For this review, take the finished solid that the model builds, in its own axes (mm). Face numbers are marked on the shaded views. A direction names the side the tool comes from. Coordinates: 2 decimals unless noted, no trailing zeros. Write each loop counter-clockwise with the first axis right and the second up, starting at its lowest first coordinate (ties: lowest second). Pieces come first, ordered by that corner, then holes. Notation, with made-up numbers: (47.5, -10) -> (71.5, -10) arc R27 ccw to (71.5, 18) -> close; hole circle Ø2 at (83.5, 70). An arc over 180 degrees is marked (long way). One line per item, written item: value. Start each with the question number.
1) Mouldability with a two-part tool opening along Y and no side actions: class the marked faces 1 and 2 as released by +Y, released by -Y, zero draft, split by the parting line, or undercut.
2) Add section B-B (z = 58). State the section outline as (x, y) points, and give its area (3 significant figures).
3) Machinability: for the marked faces 3 and 4, which of the approach directions +Z, -Z, +X, -X, +Y, -Y give a long, thin tool a straight path to every point of the face, cutting with its end or side? Answer none if there is none.
4) For pin 1 Ø6.5 at (x, z) = (0, 40.5) entering from -Y; pin 2 Ø3 at (x, z) = (-3, 58) entering from +Y; pin 3 Ø6 at (y, z) = (-4.5, 42.5) entering from -X; pin 4 Ø16 at (x, y) = (0, 0) entering from -Z, all flat-tipped, find the tip position at first contact; note any pin that passes through.
5) Add section A-A (x = 0). State the section outline as (y, z) points, and give its area (3 significant figures).
6) For probe 1 along Z at (x, y) = (1, -11); probe 2 along Y at (x, z) = (0, 68); probe 3 along Z at (x, y) = (0, 10.85), list the stretches that pass through material, from the lowest coordinate up. Write a range as from..to.
7) Add section D-D (x = 4). State the section outline as (y, z) points.
8) Add section C-C (y = 14). State the section outline as (x, z) points, and give its area (3 significant figures).
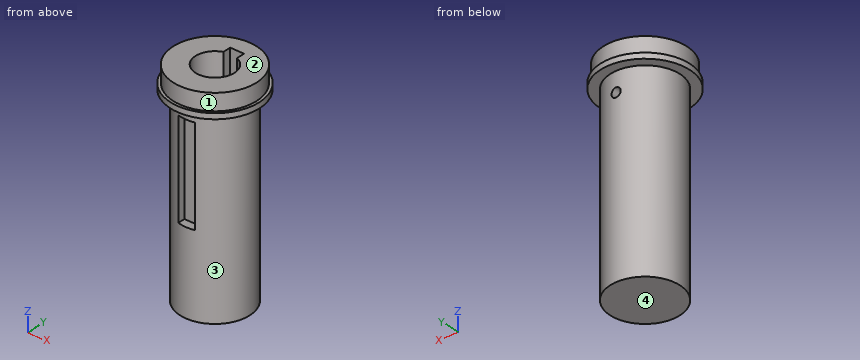
from build123d import *

# Parameters (mm, degrees)
SKETCH1_R                 = 12.5
BOSS_EXTRUDE1_DEPTH       = 68.7
SKETCH2_R                 = 16
BOSS_EXTRUDE2_DEPTH       = 2
SKETCH3_R                 = 15
BOSS_EXTRUDE3_DEPTH       = 6
CUT_EXTRUDE1_DEPTH        = 30
SKETCH6_W                 = 6
SKETCH6_H                 = 6
CUT_EXTRUDE2_DEPTH        = 35
M4X0_7_TAPPED_HOLE1_D     = 3.3
M4X0_7_TAPPED_HOLE1_DEPTH = 3


with BuildPart() as part:
    # Sketch1 → Boss-Extrude1 (new body)
    with BuildSketch(Plane.XY):
        Circle(SKETCH1_R)
    extrude(amount=BOSS_EXTRUDE1_DEPTH)

    # Sketch2 → Boss-Extrude2 (add)
    with BuildSketch(Plane.XY.offset(68.7)):
        Circle(SKETCH2_R)
    extrude(amount=BOSS_EXTRUDE2_DEPTH)

    # Sketch3 → Boss-Extrude3 (add)
    with BuildSketch(Plane.XY.offset(70.7)):
        Circle(SKETCH3_R)
    extrude(amount=BOSS_EXTRUDE3_DEPTH)

    # Sketch4 → Cut-Extrude1 (cut)
    with BuildSketch(Plane.XY.offset(76.7)):
        with BuildLine():
            Line((-2.5, 6.538348415), (-2.5, 4.5))
            Line((-2.5, 4.5), (2.5, 4.5))
            Line((2.5, 4.5), (2.5, 6.538348415))
            ThreePointArc((2.5, 6.538348415), (0, 7), (-2.5, 6.538348415))
        make_face()
        with BuildLine():
            Line((2.5, 4.5), (-2.5, 4.5))
            Line((-2.5, 4.5), (-2.5, 6.538348415))
            ThreePointArc((-2.5, 6.538348415), (-3.968626967, -5.766281297), (7, 0))
            ThreePointArc((7, 0), (5.766281297, 3.968626967), (2.5, 6.538348415))
            Line((2.5, 6.538348415), (2.5, 4.5))
        make_face()
        with BuildLine():
            Line((-2.5, 9.5), (-2.5, 6.538348415))
            ThreePointArc((-2.5, 6.538348415), (0, 7), (2.5, 6.538348415))
            Line((2.5, 6.538348415), (2.5, 9.5))
            Line((2.5, 9.5), (-2.5, 9.5))
        make_face()
    extrude(amount=-CUT_EXTRUDE1_DEPTH, mode=Mode.SUBTRACT)

    # Sketch6 → Cut-Extrude2 (cut)
    with BuildSketch(Plane(origin=(0, 0, 64.7), x_dir=(-1, 0, 0), z_dir=(0, 0, -1))):
        with Locations((0, -12.5)):
            Rectangle(SKETCH6_W, SKETCH6_H)
    extrude(amount=CUT_EXTRUDE2_DEPTH, mode=Mode.SUBTRACT)

    # M4x0.7 Tapped Hole1
    with Locations(Plane(origin=(0, 12.5, 0), x_dir=(1, 0, 0), z_dir=(0, 1, 0))):
        with Locations((0, -61.7)):
            Hole(M4X0_7_TAPPED_HOLE1_D / 2, depth=M4X0_7_TAPPED_HOLE1_DEPTH)


solid = part.part
Numbers:
1. face 1: split by the parting line
1. face 2: zero draft
2. outline: (-3, -12.13) -> (-3, -9.5) -> (3, -9.5) -> (3, -12.13) arc R12.5 ccw (long way) to start; hole (-2.5, 6.54) arc R7 ccw (long way) to (2.5, 6.54) -> (2.5, 9.5) -> (-2.5, 9.5) -> close
2. area: 306 mm²
3. face 3: -Z
3. face 4: -Z, +X, -X, +Y, -Y
4. pin 1: y = -12.13
4. pin 2: y = 12.41
4. pin 3: x = -12.41
4. pin 4: z = 0
5. outline: (-16, 68.7) -> (-12.5, 68.7) -> (-12.5, 64.7) -> (-9.5, 64.7) -> (-9.5, 29.7) -> (-12.5, 29.7) -> (-12.5, 0) -> (12.5, 0) -> (12.5, 60.05) -> (9.5, 60.05) -> (9.5, 46.7) -> (-7, 46.7) -> (-7, 76.7) -> (-15, 76.7) -> (-15, 70.7) -> (-16, 70.7) -> close; (9.5, 63.35) -> (12.5, 63.35) -> (12.5, 68.7) -> (16, 68.7) -> (16, 70.7) -> (15, 70.7) -> (15, 76.7) -> (9.5, 76.7) -> close
5. area: 1,350 mm²
6. probe 1: 0..29.7, 64.7..76.7
6. probe 2: -12.5..-7, 9.5..12.5
6. probe 3: 0..60.05, 63.35..76.7
7. outline: (-15.49, 68.7) -> (-11.84, 68.7) -> (-11.84, 0) -> (11.84, 0) -> (11.84, 68.7) -> (15.49, 68.7) -> (15.49, 70.7) -> (14.46, 70.7) -> (14.46, 76.7) -> (5.74, 76.7) -> (5.74, 46.7) -> (-5.74, 46.7) -> (-5.74, 76.7) -> (-14.46, 76.7) -> (-14.46, 70.7) -> (-15.49, 70.7) -> close
8. outline: (-7.75, 68.7) -> (7.75, 68.7) -> (7.75, 70.7) -> (5.39, 70.7) -> (5.39, 76.7) -> (-5.39, 76.7) -> (-5.39, 70.7) -> (-7.75, 70.7) -> close
8. area: 95.6 mm²
